For this review, use the dimensioned drawing (mm, ordinates from the lowest corner) and the shaded views. Coordinates: 2 decimals unless noted, no trailing zeros. Write each loop counter-clockwise with the first axis right and the second up, starting at its lowest first coordinate (ties: lowest second). Pieces come first, ordered by that corner, then holes. Notation, with made-up numbers: (45.25, 64) -> (64.25, 64) arc R29 cw to (64.25, 96) -> close; hole circle Ø1 at (86, 88.25). An arc over 180 degrees is marked (long way). Put each result on its own line as item: value. Start each with the question number.
Item 1: Consider section A-A on y = 137.16. Give the boundary of the cut face in (x, z).
Item 2: To check wall thickness, follow L1, parallel to X at y = 137.16, z = 1.85; L2, parallel to X at y = 201.93, z = 1.6; L3, parallel to Y at x = 20, z = 1.8. State the ranges of each line that lie inside material, in increasing order.
Item 3: Insertion check: P1, Ø4, axis at x = 19.431, y = 137.16, coming from the -Z side (1 decimal). The pin has a flat end and moves straight along its axis. Give the tip position at first contact, or say it passes through.
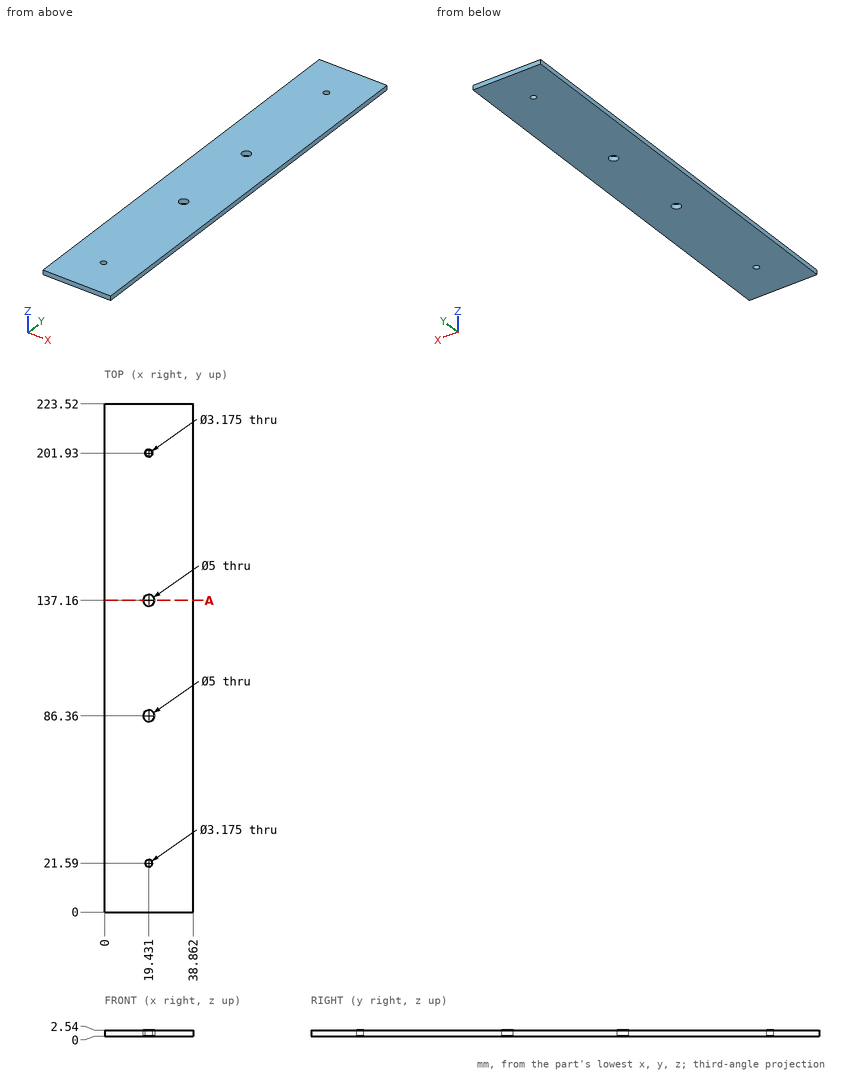
Return value:
1. outline: (0, 0) -> (16.93, 0) -> (16.93, 2.54) -> (0, 2.54) -> close; (21.93, 0) -> (38.86, 0) -> (38.86, 2.54) -> (21.93, 2.54) -> close
2. L1: 0 to 16.93, 21.93 to 38.86
2. L2: 0 to 17.84, 21.02 to 38.86
2. L3: 0 to 20.11, 23.07 to 83.93, 88.79 to 134.73, 139.59 to 200.45, 203.41 to 223.52
3. P1: through
